from build123d import *

# Parameters (mm, degrees)
SKETCH1_W           = 31.75
SKETCH1_H           = 33.02
BOSS_EXTRUDE1_DEPTH = 31.75
CUT_EXTRUDE1_START  = 3.175
SKETCH1_3_W         = 25.4
SKETCH1_3_H         = 12.7
CUT_EXTRUDE1_DEPTH  = 25.4
CUT_EXTRUDE2_START  = 9.525
CUT_EXTRUDE2_DEPTH  = 12.7


with BuildPart() as part:
    # Sketch1 → Boss-Extrude1 (new body)
    with BuildSketch(Plane.XY):
        Rectangle(SKETCH1_W, SKETCH1_H)
    extrude(amount=BOSS_EXTRUDE1_DEPTH)

    # Sketch1<3> → Cut-Extrude1 (cut)
    with BuildSketch(Plane.XY.offset(CUT_EXTRUDE1_START)):
        with Locations((0, -10.16)):
            Rectangle(SKETCH1_3_W, SKETCH1_3_H)
    extrude(amount=CUT_EXTRUDE1_DEPTH, mode=Mode.SUBTRACT)

    # Sketch1<4> → Cut-Extrude2 (cut)
    with BuildSketch(Plane.XY.offset(CUT_EXTRUDE2_START)):
        with BuildLine():
            Line((-15.875, 8.762680903), (-15.875, -3.825884934))
            ThreePointArc((-15.875, -3.825884934), (0, 3.81), (15.875, -3.825884934))
            Line((15.875, -3.825884934), (15.875, 8.762680903))
            ThreePointArc((15.875, 8.762680903), (0, 13.335), (-15.875, 8.762680903))
        make_face()
    extrude(amount=CUT_EXTRUDE2_DEPTH, mode=Mode.SUBTRACT)


solid = part.part
Build history of the part. All positions in model axes, mm. A direction names the side the tool comes from. Round coordinates to 2 decimals unless told otherwise and drop trailing zeros. Write each loop counter-clockwise with the first axis right and the second up, starting at its lowest first coordinate (ties: lowest second). Pieces come first, ordered by that corner, then holes. Notation, with made-up numbers: M 17.25,89 L 35.25,89 A18 ccw 35.25,100 Z; hole C 12.5,-25 d7. An arc over 180 degrees is marked long. Answer as a JSON object with one key per item and string values. Group by question number.
(1) Mould opens along Y. For faces 4 (the flat face through (12.7, -10, 16)), 5 (the flat face through (0, 16.51, 16)), 6 (the flat face through (0, 7, 22.225)) say: pulls with the +Y half, pulls with the -Y half, needs draft (parallel to the pull), parting line crosses it, or undercut.
(2) Cut at A-A (z = 10). Give the cut face in (x, y) (3 decimals).
(3) Cut at D-D (z = 28). Give the cut face in (x, y) (3 decimals), and give its area (3 significant figures).
(4) Cut at B-B (y = 4.5). Give the cut face in (x, z) (3 decimals), and give its area (3 significant figures).
(5) Which spindle directions (+Z, -Z, +X, -X, +Y, -Y) get a long thin tool onto all of the face, cutting with end or side? Do faces 1 (the flat face through (0, -10, 3.175)), 2 (the flat face through (0, 0, 31.75)), 3 (the flat face through (0, 7, 9.525)). Say none if no direction does.
(6) Flat gauge pin, fed straight in: pin 1 (4 mm diameter, centred on x = -5, z = 19, fed in from -Y). Where does the tip first touch, or does it go through?
(7) Cut at C-C (x = -9.5). Give the cut face in (y, z) (3 decimals), and give its area (3 significant figures).
(8) Drill centre lines: L1, parallel to Z at x = -10, y = 7.5 (3 decimals); L2, parallel to Z at x = 8, y = -14 (3 decimals); L3, parallel to X at y = -9.5, z = 15.5 (3 decimals). Where is each one in solid material? Low to high.
Responses:
{
 "1": {"face 4": "needs draft", "face 5": "pulls with the +Y half", "face 6": "undercut"},
 "2": {"outline": "M -15.875,-16.51 L -12.7,-16.51 L -12.7,-3.81 L 12.7,-3.81 L 12.7,-16.51 L 15.875,-16.51 L 15.875,-3.826 A20.32 ccw -15.875,-3.826 Z; M -15.875,8.763 A29.845 cw 15.875,8.763 L 15.875,16.51 L -15.875,16.51 Z"},
 "3": {"outline": "M -15.875,-16.51 L -12.7,-16.51 L -12.7,-3.81 L 12.7,-3.81 L 12.7,-16.51 L 15.875,-16.51 L 15.875,16.51 L -15.875,16.51 Z", "area": "726 mm2"},
 "4": {"outline": "M -15.875,0 L 15.875,0 L 15.875,9.525 L -15.875,9.525 Z; M -15.875,22.225 L 15.875,22.225 L 15.875,31.75 L -15.875,31.75 Z", "area": "605 mm2"},
 "5": {"face 1": "-Y", "face 2": "+Z, +X, -X, +Y, -Y", "face 3": "none"},
 "6": {"pin 1": "stops at y = -3.81"},
 "7": {"outline": "M -16.51,0 L 16.51,0 L 16.51,31.75 L -16.51,31.75 L -16.51,28.575 L -3.81,28.575 L -3.81,3.175 L -16.51,3.175 Z; hole M 1.453,9.525 L 11.783,9.525 L 11.783,22.225 L 1.453,22.225 Z", "area": "595 mm2"},
 "8": {"L1": "z = 0 to 9.525, 22.225 to 31.75", "L2": "z = 0 to 3.175, 28.575 to 31.75", "L3": "x = -15.875 to -12.7, 12.7 to 15.875"}
}
